from build123d import *

# Parameters (mm, degrees)
F0_W     = 43
F0_H     = 43
F1_DEPTH = 5
F2_W     = 5
F2_H     = 5
F3_DEPTH = 1


with BuildPart() as f1:
    # F0 (on Top) → F1 (new body)
    with BuildSketch(Plane.XY):
        with Locations((21.5, -21.5)):
            Rectangle(F0_W, F0_H)
    extrude(amount=F1_DEPTH)

    # F2 (on face) → F3 (cut)
    with BuildSketch(Plane.XY.offset(5)):
        with Locations((6.5, -6.5)):
            Rectangle(F2_W, F2_H)
        with Locations((6.5, -12.5)):
            Rectangle(F2_W, F2_H)
        with Locations((6.5, -18.5)):
            Rectangle(F2_W, F2_H)
        with Locations((6.5, -24.5)):
            Rectangle(F2_W, F2_H)
        with Locations((18.5, -6.5)):
            Rectangle(F2_W, F2_H)
        with Locations((18.5, -12.5)):
            Rectangle(F2_W, F2_H)
        with Locations((18.5, -18.5)):
            Rectangle(F2_W, F2_H)
        with Locations((30.5, -24.5)):
            Rectangle(F2_W, F2_H)
        with Locations((30.5, -30.5)):
            Rectangle(F2_W, F2_H)
        with Locations((30.5, -36.5)):
            Rectangle(F2_W, F2_H)
        with Locations((36.5, -6.5)):
            Rectangle(F2_W, F2_H)
        with Locations((36.5, -12.5)):
            Rectangle(F2_W, F2_H)
        with Locations((36.5, -18.5)):
            Rectangle(F2_W, F2_H)
        with Locations((36.5, -36.5)):
            Rectangle(F2_W, F2_H)
        with Locations((36.5, -30.5)):
            Rectangle(F2_W, F2_H)
        with Locations((36.5, -24.5)):
            Rectangle(F2_W, F2_H)
        with Locations((30.5, -18.5)):
            Rectangle(F2_W, F2_H)
        with Locations((30.5, -12.5)):
            Rectangle(F2_W, F2_H)
        with Locations((30.5, -6.5)):
            Rectangle(F2_W, F2_H)
        with Locations((24.5, -36.5)):
            Rectangle(F2_W, F2_H)
        with Locations((24.5, -30.5)):
            Rectangle(F2_W, F2_H)
        with Locations((24.5, -24.5)):
            Rectangle(F2_W, F2_H)
        with Locations((24.5, -18.5)):
            Rectangle(F2_W, F2_H)
        with Locations((24.5, -12.5)):
            Rectangle(F2_W, F2_H)
        with Locations((24.5, -6.5)):
            Rectangle(F2_W, F2_H)
        with Locations((18.5, -36.5)):
            Rectangle(F2_W, F2_H)
        with Locations((18.5, -30.5)):
            Rectangle(F2_W, F2_H)
        with Locations((12.5, -36.5)):
            Rectangle(F2_W, F2_H)
        with Locations((6.5, -36.5)):
            Rectangle(F2_W, F2_H)
        with Locations((6.5, -30.5)):
            Rectangle(F2_W, F2_H)
        with Locations((12.5, -30.5)):
            Rectangle(F2_W, F2_H)
        with Locations((12.5, -24.5)):
            Rectangle(F2_W, F2_H)
        with Locations((18.5, -24.5)):
            Rectangle(F2_W, F2_H)
        with Locations((12.5, -18.5)):
            Rectangle(F2_W, F2_H)
        with Locations((12.5, -12.5)):
            Rectangle(F2_W, F2_H)
        with Locations((12.5, -6.5)):
            Rectangle(F2_W, F2_H)
    extrude(amount=-F3_DEPTH, mode=Mode.SUBTRACT)


solid = f1.part
Model file for the job. Use its own axes, mm. Give positions to 0.01 mm unless a question says otherwise; leave off trailing zeros. Loops run counter-clockwise (first coordinate to the right, second up) from the corner with the lowest first, then second, coordinate; pieces in that order, holes last.
1) Wall check: line 1 (Z direction, x = 29, y = -36). Give the ranges that are in metal, low to high.
2) Pull direction X, two halves, no side cores. Call faces 1 (the flat face through (6.5, -15, 4.5)), 2 (the flat face through (21, 0, 2)): +X half, -X half, draft (parallel to the pull), parting line (faces both ways), or undercut.
3) Saw through at B-B (x = 11). Write the cut outline in (y, z), plus the area to 3 significant figures.
4) Saw through at A-A (y = -23.5). Write the cut outline in (x, z).
Answer block:
1. line 1: z = 0 to 4
2. face 1: undercut
2. face 2: draft
3. outline: (-43, 0) - (0, 0) - (0, 5) - (-4, 5) - (-4, 4) - (-9, 4) - (-9, 5) - (-10, 5) - (-10, 4) - (-15, 4) - (-15, 5) - (-16, 5) - (-16, 4) - (-21, 4) - (-21, 5) - (-22, 5) - (-22, 4) - (-27, 4) - (-27, 5) - (-28, 5) - (-28, 4) - (-33, 4) - (-33, 5) - (-34, 5) - (-34, 4) - (-39, 4) - (-39, 5) - (-43, 5) - close
3. area: 185 mm2
4. outline: (0, 0) - (43, 0) - (43, 5) - (39, 5) - (39, 4) - (34, 4) - (34, 5) - (33, 5) - (33, 4) - (28, 4) - (28, 5) - (27, 5) - (27, 4) - (22, 4) - (22, 5) - (21, 5) - (21, 4) - (16, 4) - (16, 5) - (15, 5) - (15, 4) - (10, 4) - (10, 5) - (9, 5) - (9, 4) - (4, 4) - (4, 5) - (0, 5) - close
